Autodesk Inventor part; units mm, degrees
ref_plane "YZ Plane" through (0, 0, 0) normal (1, 0, 0) x (0, 1, 0)
ref_plane "XZ Plane" through (0, 0, 0) normal (0, 1, 0) x (-1, 0, 0)
ref_plane "XY Plane" through (0, 0, 0) normal (0, 0, 1) x (1, 0, 0)
sketch "Sketch1" plane through (0, 0, 0) normal (0, 1, 0) x (-1, 0, 0)
  circle A0 centre (29.9915, -10) radius 2.75
  circle A1 centre (9.9915, -10) radius 2.75
  line L0 (0, 0) -> (0, -6.5)
  line L1 (-0.0085, -20) -> (-0.0085, -13.5)
  line L2 (0, -6.5) -> (0.5, -6.5)
  line L3 (0.5, -6.5) -> (0.5, -7)
  line L4 (0.5, -7) -> (1, -7)
  line L5 (-0.0085, -13.5) -> (0.4915, -13.5)
  line L6 (0.4915, -13.5) -> (0.4915, -13)
  line L7 (0.4915, -13) -> (0.9915, -13)
  line L8 (1, -4.05) -> (3, -4.05)
  line L9 (0.9915, -15.95) -> (2.9915, -15.95)
  line L10 (5.5, -6.5) -> (5.5, -13.5)
  line L11 (5.5, -13.5) -> (2.9915, -15.95)
  line L12 (5.5, -6.5) -> (3, -4.05)
  line L13 (1, -4.05) -> (1, -7)
  line L14 (0.9915, -13) -> (0.9915, -15.95)
  line L15 (-0.0085, -20) -> (6.4915, -20)
  line L16 (6.4915, -20) -> (6.4915, -19.5)
  line L17 (6.4915, -19.5) -> (6.9915, -19.5)
  line L18 (6.9915, -19.5) -> (6.9915, -19)
  line L19 (6.9915, -19) -> (4.0415, -19)
  line L20 (4.0415, -19) -> (4.0415, -17)
  line L21 (13.4915, -20) -> (13.4915, -19.5)
  line L22 (13.4915, -19.5) -> (12.9915, -19.5)
  line L23 (12.9915, -19.5) -> (12.9915, -19)
  line L24 (12.9915, -19) -> (15.9415, -19)
  line L25 (15.9415, -19) -> (15.9415, -17)
  line L26 (15.9415, -17) -> (13.4915, -14.5)
  line L27 (6.4915, -14.5) -> (13.4915, -14.5)
  line L28 (4.0415, -17) -> (6.4915, -14.5)
  line L29 (39.9915, 0) -> (39.9915, -6.5)
  line L30 (39.9915, -6.5) -> (39.4915, -6.5)
  line L31 (39.4915, -6.5) -> (39.4915, -7)
  line L32 (39.4915, -7) -> (38.9915, -7)
  line L33 (38.9915, -7) -> (38.9915, -4.05)
  line L34 (38.9915, -4.05) -> (36.9915, -4.05)
  line L35 (39.9915, -20) -> (39.9915, -13.5)
  line L36 (39.9915, -13.5) -> (39.4915, -13.5)
  line L37 (39.4915, -13.5) -> (39.4915, -13)
  line L38 (39.4915, -13) -> (38.9915, -13)
  line L39 (38.9915, -13) -> (38.9915, -15.95)
  line L40 (38.9915, -15.95) -> (36.9915, -15.95)
  line L41 (34.4915, -6.601) -> (34.4915, -13.5)
  line L42 (34.4915, -13.5) -> (36.9915, -15.95)
  line L43 (34.4915, -6.601) -> (36.9915, -4.05)
  line L44 (39.9915, -20) -> (33.4915, -20)
  line L45 (33.4915, -20) -> (33.4915, -19.5)
  line L46 (33.4915, -19.5) -> (32.9915, -19.5)
  line L47 (32.9915, -19.5) -> (32.9915, -19)
  line L48 (32.9915, -19) -> (35.9415, -19)
  line L49 (35.9415, -19) -> (35.9415, -17)
  line L50 (26.4915, -20) -> (26.4915, -19.5)
  line L51 (26.4915, -19.5) -> (26.9915, -19.5)
  line L52 (26.9915, -19.5) -> (26.9915, -19)
  line L53 (26.9915, -19) -> (24.0415, -19)
  line L54 (24.0415, -19) -> (24.0415, -17)
  line L55 (33.4915, -14.5) -> (26.4915, -14.5)
  line L56 (24.0415, -17) -> (26.4915, -14.5)
  line L57 (33.4915, -14.5) -> (35.9415, -17)
  line L58 (26.4915, -20) -> (13.4915, -20)
  line L59 (39.9915, 0) -> (33.4915, 0)
  line L60 (33.4915, 0) -> (33.4915, -0.5)
  line L61 (33.4915, -0.5) -> (32.9915, -0.5)
  line L62 (32.9915, -0.5) -> (32.9915, -1)
  line L63 (32.9915, -1) -> (35.9415, -1)
  line L64 (35.9415, -1) -> (35.9415, -3)
  line L65 (26.4915, 0) -> (26.4915, -0.5)
  line L66 (26.4915, -0.5) -> (26.9915, -0.5)
  line L67 (26.9915, -0.5) -> (26.9915, -1)
  line L68 (26.9915, -1) -> (24.0415, -1)
  line L69 (24.0415, -1) -> (24.0415, -3)
  line L70 (33.4915, -5.5) -> (26.4915, -5.5)
  line L71 (24.0415, -3) -> (26.4915, -5.5)
  line L72 (35.9415, -3) -> (33.4915, -5.5)
  line L73 (0, 0) -> (6.5, 0)
  line L74 (6.5, 0) -> (6.5, -0.5)
  line L75 (6.5, -0.5) -> (7, -0.5)
  line L76 (7, -0.5) -> (7, -1)
  line L77 (7, -1) -> (4.05, -1)
  line L78 (4.05, -1) -> (4.05, -3)
  line L79 (13.5, 0) -> (13.5, -0.5)
  line L80 (13.5, -0.5) -> (13, -0.5)
  line L81 (13, -0.5) -> (13, -1)
  line L82 (13, -1) -> (15.95, -1)
  line L83 (15.95, -1) -> (15.95, -3)
  line L84 (13.5, -5.5) -> (6.5, -5.5)
  line L85 (6.5, -5.5) -> (4.05, -3)
  line L86 (15.95, -3) -> (13.5, -5.5)
  line L87 (13.5, 0) -> (26.4915, 0)
  dimension "d0" = 40
  dimension "d1" = 20
  dimension "d2" = 5.5
  dimension "d3" = 5.5
  dimension "d4" = 20
  dimension "d11" = 6.5
  dimension "d12" = 6.5
  dimension "d13" = 0.5
  dimension "d14" = 0.5
  dimension "d15" = 0.5
  dimension "d16" = 0.5
  dimension "d17" = 0.5
  dimension "d18" = 0.5
  dimension "d19" = 5.5
  dimension "d20" = 11.9
  dimension "d21" = 6.5
  dimension "d22" = 0.5
  dimension "d23" = 0.5
  dimension "d24" = 0.5
  dimension "d25" = 0.5
  dimension "d26" = 0.5
  dimension "d27" = 0.5
  dimension "d28" = 7
  dimension "d29" = 11.9
  dimension "d31" = 4.05
  dimension "d32" = 2.95
  dimension "d34" = 2
  dimension "d35" = 2
  dimension "d36" = 2
  dimension "d37" = 2
  dimension "d39" = 7
  dimension "d40" = 6.5
  dimension "d41" = 0.5
  dimension "d42" = 0.5
  dimension "d43" = 0.5
  dimension "d44" = 2.95
  dimension "d45" = 2
  dimension "d46" = 6.5
  dimension "d47" = 0.5
  dimension "d48" = 0.5
  dimension "d49" = 0.5
  dimension "d50" = 2.95
  dimension "d51" = 2
  dimension "d52" = 5.5
  dimension "d53" = 6.5
  dimension "d54" = 0.5
  dimension "d55" = 0.5
  dimension "d56" = 0.5
  dimension "d57" = 2.95
  dimension "d58" = 2
  dimension "d59" = 0.5
  dimension "d60" = 0.5
  dimension "d61" = 0.5
  dimension "d62" = 2.95
  dimension "d63" = 2
  dimension "d64" = 7
  dimension "d66" = 6.5
  dimension "d67" = 0.5
  dimension "d68" = 0.5
  dimension "d69" = 0.5
  dimension "d70" = 2.95
  dimension "d71" = 2
  dimension "d72" = 0.5
  dimension "d73" = 0.5
extrude "Extrusion1" add sketch "Sketch1" along normal blind 965.2
properties part number "Tslot_2040extrusion_38inch"
Check sheet for the modelled part. Datum: model origin and axes. Units: mm. Coordinates: 2 decimals unless noted, no trailing zeros. Answer in a Markdown table with one row per item.
1. Sectioned sample at A-A, the plane y = 483.5. Give the number of separate pieces and of enclosed holes in the cut face, then the cut area to 3 significant figures.
Check values:
| item | result |
|---|---|
| separate pieces | 1 |
| enclosed holes | 2 |
| area | 429 mm2 |
2. Material ranges on line 1 along X through (y, z) = (624.5, -18.5); line 2 along Z through (x, y) = (-25, 814); line 3 along X through (y, z) = (724.5, -9.75), recorded low to high. Write a range as [from, to].
Check values:
| item | result |
|---|---|
| line 1 | x = [-39.99, -35.94], [-24.04, -15.94], [-4.04, 0.01] |
| line 2 | z = [-20, -19], [-16.02, -3.98], [-1, 0] |
| line 3 | x = [-34.49, -32.73], [-27.25, -12.73], [-7.25, -5.5] |
3. Go/stop test with flat-tipped pins: pin 1 (1.5 mm diameter, centred on y = 863, z = -6, fed in from +X); pin 2 (4.5 mm diameter, centred on x = -29.99, z = -10, fed in from -Y). Record where each tip stops, or that it passes through.
Check values:
| item | result |
|---|---|
| pin 1 | stops at x = 0 |
| pin 2 | passes through |
